Source: CAD feature listing. Evaluate the final solid. Frame: model axes, mm. A direction names the side the tool comes from. Coordinates: 2 decimals unless noted, no trailing zeros. Write each loop counter-clockwise with the first axis right and the second up, starting at its lowest first coordinate (ties: lowest second). Pieces come first, ordered by that corner, then holes. Notation, with made-up numbers: (62, -33) -> (111, -33) arc R20 cw to (111, 1) -> close; hole circle Ø1 at (55.5, 34). An arc over 180 degrees is marked (long way). One line per item, written item: value. Start each with the question number.
1. Mould query, pull axis X, two halves, no side actions, for faces 3 (the flat face through (14.85, 0, 7)), 4 (the cylindrical face through (0.802, -3.612, 0.986)), 5 (the cylindrical face through (-13.86, 6.08, 6.15)), 6 (the flat face through (3, 3, 2)). Classes: released by +X, released by -X, zero draft, split by the parting line, or undercut.
2. Section query D-D, the plane y = 0. Output: boundary loops of the cut face in (x, z), and give its area (3 significant figures).
3. Section query B-B, the plane z = 19.5. Output: boundary loops of the cut face in (x, y), and give its area (3 significant figures).
4. First-contact query: P1, Ø4.5, axis at x = -6, y = -6, coming from the +Z side; P2, Ø2, axis at x = 13.5, y = -1, coming from the +Z side; P3, Ø5, axis at y = -5, z = 19.5, coming from the +X side. Flat tips, straight axial feed; report the tip coordinate or a pass-through.
5. Access query for faces 1 (the flat face through (-14.85, 0, 13)), 2 (the flat face through (12.85, 0, 8)). Directions: +Z, -Z, +X, -X, +Y, -Y. A direction counts if a zero-diameter tool reaches every point of the face in a straight line with its end or side. Return the directions, or none.
6. Line query: line 1 (Y direction, x = -6, z = 1.3); line 2 (X direction, y = -4.5, z = 6.75); line 3 (Z direction, x = -10.25, y = 6). Output: solid intervals per line, ascending.
7. Section query C-C, the plane x = -6. Output: boundary loops of the cut face in (y, z).
8. Section query A-A, the plane y = -6. State how many separate pieces and enclosed holes the cut face has, and give its area (3 significant figures).
from build123d import *

# Parameters (mm, degrees)
BOSS_EXTRUDE1_DEPTH = 12.7
SKETCH2_R           = 1.85
CUT_EXTRUDE1_DEPTH  = 30.7
SKETCH3_R           = 3.7
CUT_EXTRUDE2_DEPTH  = 15
SKETCH4_R           = 1.85
CUT_EXTRUDE3_DEPTH  = 3
SKETCH5_W           = 11.5
SKETCH5_H           = 25.4
SKETCH5_R           = 1.85
BOSS_EXTRUDE2_DEPTH = 2
FILLET1_R           = 1


with BuildPart() as part:
    # Sketch1 → Boss-Extrude1 (new body, symmetric)
    with BuildSketch(Plane(origin=(0, 0, 0), x_dir=(1, 0, 0), z_dir=(0, 1, 0))):
        Polygon((-14.85, 0), (14.85, 0), (14.85, -14), (12.85, -14), (12.85, -2), (-12.85, -2), (-12.85, -14), (-14.85, -14), align=None)
    extrude(amount=BOSS_EXTRUDE1_DEPTH, both=True)

    # Sketch2 → Cut-Extrude1 (cut, through all)
    with BuildSketch(Plane.ZY.offset(14.85)):
        with Locations((8, -6)):
            Circle(SKETCH2_R)
        with Locations((8, 6)):
            Circle(SKETCH2_R)
    extrude(amount=-CUT_EXTRUDE1_DEPTH, mode=Mode.SUBTRACT)

    # Sketch3 → Cut-Extrude2 (cut, through all)
    with BuildSketch(Plane(origin=(0, 0, 0), x_dir=(-1, 0, 0), z_dir=(0, 0, -1))):
        Circle(SKETCH3_R)
    extrude(amount=-CUT_EXTRUDE2_DEPTH, mode=Mode.SUBTRACT)

    # Sketch4 → Cut-Extrude3 (cut, through all)
    with BuildSketch(Plane.XY.offset(2)):
        with Locations((-6, 6)):
            Circle(SKETCH4_R)
        with Locations((-6, -6)):
            Circle(SKETCH4_R)
        with Locations((6, -6)):
            Circle(SKETCH4_R)
        with Locations((6, 6)):
            Circle(SKETCH4_R)
    extrude(amount=-CUT_EXTRUDE3_DEPTH, mode=Mode.SUBTRACT)

    # Sketch5 → Boss-Extrude2 (add)
    with BuildSketch(Plane(origin=(-14.85, 0, 0), x_dir=(0, 0, -1), z_dir=(1, 0, 0))):
        with Locations((-19.75, 0)):
            Rectangle(SKETCH5_W, SKETCH5_H)
        with Locations((-19.5, 6)):
            Circle(SKETCH5_R, mode=Mode.SUBTRACT)
        with Locations((-19.5, -6)):
            Circle(SKETCH5_R, mode=Mode.SUBTRACT)
    extrude(amount=BOSS_EXTRUDE2_DEPTH)

    # Fillet1
    fillet1_edges = [part.edges().sort_by_distance(p)[0] for p in [
        (-14.85, 0, 0),
        (14.85, 0, 0),
    ]]
    fillet(fillet1_edges, radius=FILLET1_R)


solid = part.part
Computed values:
1. face 3: released by +X
1. face 4: undercut
1. face 5: zero draft
1. face 6: undercut
2. outline: (-14.85, 1) arc R1 ccw to (-13.85, 0) -> (-3.7, 0) -> (-3.7, 2) -> (-12.85, 2) -> (-12.85, 25.5) -> (-14.85, 25.5) -> close; (3.7, 0) -> (13.85, 0) arc R1 ccw to (14.85, 1) -> (14.85, 14) -> (12.85, 14) -> (12.85, 2) -> (3.7, 2) -> close
2. area: 115 mm²
3. outline: (-14.85, -12.7) -> (-12.85, -12.7) -> (-12.85, -7.85) -> (-14.85, -7.85) -> close; (-14.85, -4.15) -> (-12.85, -4.15) -> (-12.85, 4.15) -> (-14.85, 4.15) -> close; (-14.85, 7.85) -> (-12.85, 7.85) -> (-12.85, 12.7) -> (-14.85, 12.7) -> close
3. area: 36.0 mm²
4. P1: stops at z = 2
4. P2: stops at z = 14
4. P3: stops at x = -12.85
5. face 1: +Z, -Z, -X, +Y, -Y
5. face 2: +Z, +Y, -Y
6. line 1: y = -12.7 to -7.85, -4.15 to 4.15, 7.85 to 12.7
6. line 2: x = -14.85 to -12.85, 12.85 to 14.85
6. line 3: z = 0 to 2
7. outline: (-12.7, 0) -> (-7.85, 0) -> (-7.85, 2) -> (-12.7, 2) -> close; (-4.15, 0) -> (4.15, 0) -> (4.15, 2) -> (-4.15, 2) -> close; (7.85, 0) -> (12.7, 0) -> (12.7, 2) -> (7.85, 2) -> close
8. separate pieces: 6
8. enclosed holes: 0
8. area: 93.0 mm²
